Autodesk Inventor part; units mm, degrees
ref_plane "YZ Plane" through (0, 0, 0) normal (1, 0, 0) x (0, 1, 0)
ref_plane "XZ Plane" through (0, 0, 0) normal (0, 1, 0) x (-1, 0, 0)
ref_plane "XY Plane" through (0, 0, 0) normal (0, 0, 1) x (1, 0, 0)
sketch "Sketch1" plane through (0, 0, 0) normal (0, 0, 1) x (1, 0, 0)
  line L0 (-21.2294, -12.5998) -> (21.2706, -12.5998)
  line L1 (23.2706, -10.5998) -> (23.2706, -4.1998)
  line L2 (-23.2294, -4.1998) -> (-23.2294, -10.5998)
  line L3 (12.0206, -0.1998) -> (12.0206, 21.8002)
  line L4 (10.0206, 23.8002) -> (-9.9794, 23.8002)
  line L5 (-11.9794, 21.8002) -> (-11.9794, -0.1998)
  circle A0 centre (16.0206, -7.3998) radius 1.6
  circle A1 centre (-15.9794, -7.3998) radius 1.6
  line L6 (21.2706, -2.1998) -> (14.0206, -2.1998)
  line L7 (-13.9794, -2.1998) -> (-21.2294, -2.1998)
  line L8 (0.0206, 11.8002) -> (-1.5294, 11.8002)
  line L9 (-1.5294, 11.8002) -> (1.5706, 11.8002)
  line L10 (-1.5294, 11.8002) -> (-1.5294, 13.8002)
  line L11 (-1.5294, 13.8002) -> (-2.7282, 13.8002)
  line L12 (2.7718, 13.8002) -> (2.7718, 15.8002)
  line L13 (-2.7282, 15.8002) -> (-2.7282, 13.8002)
  line L14 (-2.7282, 15.8002) -> (-1.5294, 15.8002)
  line L15 (0.0206, 15.8002) -> (0.0218, 15.8002)
  line L16 (2.7718, 15.8002) -> (1.5706, 15.8002)
  line L17 (-1.5294, 15.8002) -> (-2.7282, 15.8002)
  line L18 (-1.5294, 11.8002) -> (-1.5294, 13.8002)
  line L19 (-1.5294, 15.8002) -> (-1.5294, 23.8002)
  line L20 (-2.7282, 13.8002) -> (-1.5294, 13.8002)
  line L21 (1.5706, 13.8002) -> (2.7718, 13.8002)
  line L22 (1.5706, 11.8002) -> (1.5706, 13.8002)
  line L23 (1.5706, 15.8002) -> (1.5706, 23.8002)
  arc A2 (23.2706, -4.1998) -> (21.2706, -2.1998) centre (21.2706, -4.1998) ccw
  arc A3 (21.2706, -12.5998) -> (23.2706, -10.5998) centre (21.2706, -10.5998) ccw
  arc A4 (-23.2294, -10.5998) -> (-21.2294, -12.5998) centre (-21.2294, -10.5998) ccw
  arc A5 (-21.2294, -2.1998) -> (-23.2294, -4.1998) centre (-21.2294, -4.1998) ccw
  arc A6 (-13.9794, -2.1998) -> (-11.9794, -0.1998) centre (-13.9794, -0.1998) ccw
  arc A7 (12.0206, -0.1998) -> (14.0206, -2.1998) centre (14.0206, -0.1998) ccw
  arc A8 (-9.9794, 23.8002) -> (-11.9794, 21.8002) centre (-9.9794, 21.8002) ccw
  arc A9 (12.0206, 21.8002) -> (10.0206, 23.8002) centre (10.0206, 21.8002) ccw
  point P0 (0, 0)
  point P1 (0, 0)
  point P2 (12.0206, 23.8002)
  point P3 (-11.9794, 23.8002)
  dimension "d0" = 24
  dimension "d1" = 3.2
  dimension "d2" = 3.2
  dimension "d3" = 2
extrude "Extrusion1" add sketch "Sketch1" along normal blind 6 contours A4 L2 A5 L7 A6 L5 A8 L4 L19 L14 L13 L11 L10 L8 L9 L22 L21 L12 L16 L23 A9 L3 A7 L6 A2 L1 A3 L0
sketch "Sketch2" plane through (0, 0, 6) normal (0, 0, 1) x (1, 0, 0)
  circle A0 centre (-6.9812, 28.6469) radius 1.6
  circle A1 centre (7.0188, 28.6469) radius 1.6
  circle A2 centre (-17.6062, 13.3479) radius 1.6
  circle A3 centre (17.6438, 13.3479) radius 1.6
  line L0 (-23.2312, 26.8921) -> (-23.2312, -30.3531)
  arc A4 (-23.2312, -30.3531) -> (-21.2312, -32.3531) centre (-21.2312, -30.3531) ccw
  line L1 (-21.2312, -32.3531) -> (-7.8931, -32.3531)
  arc A5 (21.2688, -32.3531) -> (23.2688, -30.3531) centre (21.2688, -30.3531) ccw
  line L2 (23.2688, -30.3531) -> (23.2688, 26.8921)
  arc A6 (23.2688, 26.8921) -> (21.8599, 27.8047) centre (22.2688, 26.8921) ccw
  arc A7 (12.0188, 33.6469) -> (21.8599, 27.8047) centre (18.9975, 34.1927) ccw
  line L3 (12.0188, 33.6469) -> (12.0188, 39.5469)
  arc A8 (12.0188, 39.5469) -> (10.0188, 41.5469) centre (10.0188, 39.5469) ccw
  line L4 (10.0188, 41.5469) -> (2.5188, 41.5469)
  arc A9 (2.5188, 41.5469) -> (1.5188, 40.5469) centre (2.5188, 40.5469) ccw
  line L5 (1.5188, 40.5469) -> (1.5188, 36.5469)
  line L6 (1.5188, 36.5469) -> (2.7688, 36.5469)
  line L7 (2.7688, 36.5469) -> (2.7688, 33.6469)
  line L8 (2.7688, 33.6469) -> (1.5688, 33.6469)
  line L9 (1.5688, 33.6469) -> (1.5688, 23.6469)
  line L10 (1.5688, 23.6469) -> (10.0188, 23.6469)
  arc A10 (12.0188, 21.6469) -> (10.0188, 23.6469) centre (10.0188, 21.6469) ccw
  line L11 (12.0188, 21.6469) -> (12.0188, -0.3531)
  arc A11 (12.0188, -0.3531) -> (14.0188, -2.3531) centre (14.0188, -0.3531) ccw
  line L12 (14.0206, -2.3531) -> (16.2688, -2.3531)
  arc A12 (18.2688, -4.3531) -> (16.2688, -2.3531) centre (16.2688, -4.3531) ccw
  line L13 (18.2688, -4.3531) -> (18.2688, -21.3531)
  arc A13 (16.2688, -23.3531) -> (18.2688, -21.3531) centre (16.2688, -21.3531) ccw
  line L14 (16.2688, -23.3531) -> (-16.2312, -23.3531)
  arc A14 (-18.2312, -21.3531) -> (-16.2312, -23.3531) centre (-16.2312, -21.3531) ccw
  line L15 (-18.2312, -21.3531) -> (-18.2312, -4.3531)
  arc A15 (-16.2312, -2.3531) -> (-18.2312, -4.3531) centre (-16.2312, -4.3531) ccw
  line L16 (-16.2312, -2.3531) -> (-13.9794, -2.3531)
  arc A16 (-13.9794, -2.3531) -> (-11.9812, -0.5065) centre (-13.9753, -0.3531) ccw
  line L17 (-11.9812, -0.5065) -> (-11.9812, 21.4935)
  arc A17 (-9.9812, 23.4935) -> (-11.9812, 21.4935) centre (-9.9812, 21.4935) ccw
  line L18 (-9.9812, 23.4935) -> (-1.5312, 23.4935)
  line L19 (-1.5312, 23.4935) -> (-1.5312, 33.4935)
  line L20 (-1.5312, 33.4935) -> (-2.7312, 33.4935)
  line L21 (-2.7312, 33.4935) -> (-2.7312, 36.3935)
  line L22 (-2.7312, 36.3935) -> (-1.4812, 36.3935)
  line L23 (-1.4812, 36.3935) -> (-1.4812, 40.5469)
  arc A18 (-1.4812, 40.5469) -> (-2.4812, 41.5469) centre (-2.4812, 40.5469) ccw
  line L24 (-2.4812, 41.5469) -> (-9.9812, 41.5469)
  arc A19 (-9.9812, 41.5469) -> (-11.9812, 39.5469) centre (-9.9812, 39.5469) ccw
  line L25 (-11.9812, 39.5469) -> (-11.9812, 33.6469)
  arc A20 (-21.8223, 27.8047) -> (-11.9812, 33.6469) centre (-18.9599, 34.1927) ccw
  arc A21 (-21.8223, 27.8047) -> (-23.2312, 26.8921) centre (-22.2312, 26.8921) ccw
  line L26 (-13.9794, -2.3531) -> (-21.2294, -2.3531)
  arc A22 (-21.2294, -2.3531) -> (-23.2294, -4.3531) centre (-21.2294, -4.3531) ccw
  line L27 (-23.2294, -4.3531) -> (-23.2294, -10.7531)
  arc A23 (-23.2294, -10.7531) -> (-21.2294, -12.7531) centre (-21.2294, -10.7531) ccw
  line L28 (-21.2294, -12.7531) -> (21.2706, -12.7531)
  line L29 (21.2706, -2.3531) -> (14.0206, -2.3531)
  arc A24 (23.2706, -4.3531) -> (21.2706, -2.3531) centre (21.2706, -4.3531) ccw
  line L30 (23.2706, -10.7531) -> (23.2706, -4.3531)
  arc A25 (21.2706, -12.7531) -> (23.2706, -10.7531) centre (21.2706, -10.7531) ccw
  arc A26 (5.9613, -30.7014) -> (7.9307, -32.3531) centre (7.9307, -30.3531) ccw
  line L31 (7.9307, -32.3531) -> (21.2688, -32.3531)
  arc A27 (-7.8931, -32.3531) -> (-5.9236, -30.7014) centre (-7.8931, -30.3531) ccw
  arc A28 (5.9613, -30.7014) -> (-5.9236, -30.7014) centre (0.0188, -31.7522) ccw
  point P0 (0, 0)
  point P1 (-18.2312, -12.7531)
  point P2 (18.2688, -12.7531)
extrude "Extrusion2" cut sketch "Sketch2" against normal blind 6 contours A22 L26 A15 L15 L28 A23 L0 | L13 A12 L29 A24 L2 A25 L28
fillet "Fillet1" radius 2 2 edges at (18.2688, -12.5998, 3) (-18.2312, -12.5998, 3)
sketch "Sketch4" plane through (-1.5294, 11.8002, 0) normal (0, 1, 0) x (1, 0, 0)
  line L0 (3.1, 0) -> (0, 0)
  line L1 (0, 0) -> (0, -6)
  line L2 (3.1, -6) -> (0, -6)
  line L3 (3.1, 0) -> (3.1, -6)
  point P0 (1.5294, 0)
extrude "Extrusion3" cut sketch "Sketch4" against normal blind 13
sketch "Sketch5" plane through (-2.7282, 15.8002, 0) normal (0, -1, 0) x (1, 0, 0)
  line L0 (0, 0) -> (1.1988, 0)
  line L1 (1.1988, 0) -> (1.1988, 6)
  line L2 (0, 6) -> (1.1988, 6)
  line L3 (0, 0) -> (0, 6)
  line L4 (4.2988, 0) -> (5.5, 0)
  line L5 (5.5, 0) -> (5.5, 6)
  line L6 (4.2988, 6) -> (5.5, 6)
  line L7 (4.2988, 0) -> (4.2988, 6)
  point P0 (2.7282, 0)
extrude "Extrusion4" add sketch "Sketch5" along normal blind 0.4
sketch "Sketch6" plane through (0, 0, 6) normal (0, 0, 1) x (1, 0, 0)
  line L0 (22.9743, 18.6641) -> (86.0826, 18.6641) construction
  line L1 (86.0826, 18.6641) -> (86.0826, -0.0954) construction
  line L2 (86.0826, -0.0954) -> (22.9743, -0.0954) construction
  line L3 (22.9743, -0.0954) -> (22.9743, 18.6641) construction
  point P0 (0, 0)
extrude "Extrusion5" [suppressed]
properties part number "Hotend Slide Part 1"
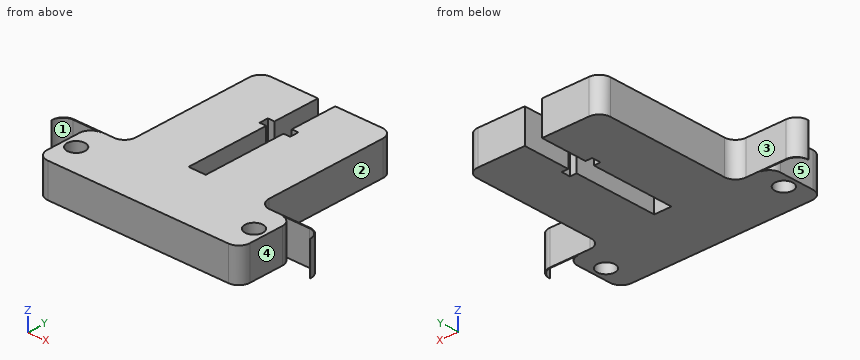
Check sheet for the modelled part. Datum: model origin and axes. Units: mm. Face numbers are marked on the shaded views. A direction names the side the tool comes from. Round coordinates to 2 decimals unless told otherwise and drop trailing zeros. Loops run counter-clockwise (first coordinate to the right, second up) from the corner with the lowest first, then second, coordinate; pieces in that order, holes last. Notation, with made-up numbers: M 10.5,13 L 63.5,13 A22 cw 63.5,28 Z; hole C 76,62.5 d5. An arc over 180 degrees is marked long. Answer as a JSON object with one key per item and string values.
1. Scan lines: line 1 (X direction, y = -7.5, z = 1.9); line 2 (X direction, y = 8, z = 4.65); line 3 (X direction, y = 14, z = 4). Record each from-to range of solid material in increasing order.
Reply:
{"line 1": "x = -18.23 to -17.58, -14.38 to 14.42, 17.62 to 18.27", "line 2": "x = -11.98 to -1.53, 1.57 to 12.02", "line 3": "x = -11.98 to -2.73, 2.77 to 12.02"}
2. Section check D-D (x = -1). Record the boundary of the cut face in (y, z).
Reply:
{"outline": "M -12.6,0 L -1.2,0 L -1.2,6 L -12.6,6 Z"}
3. Section check C-C (y = 14.5). Record the boundary of the cut face in (x, z).
Reply:
{"outline": "M -11.98,0 L -2.73,0 L -2.73,6 L -11.98,6 Z; M 2.77,0 L 12.02,0 L 12.02,6 L 2.77,6 Z"}
4. Section check B-B (y = -8). Record the boundary of the cut face in (x, z), plus the area to 3 significant figures.
Reply:
{"outline": "M -18.23,0 L -17.46,0 L -17.46,6 L -18.23,6 Z; M -14.5,0 L 14.54,0 L 14.54,6 L -14.5,6 Z; M 17.5,0 L 18.27,0 L 18.27,6 L 17.5,6 Z", "area": "183 mm²"}
5. Section check A-A (y = 3.5). Record the boundary of the cut face in (x, z), plus the area to 3 significant figures.
Reply:
{"outline": "M -11.98,0 L -1.53,0 L -1.53,6 L -11.98,6 Z; M 1.57,0 L 12.02,0 L 12.02,6 L 1.57,6 Z", "area": "125 mm²"}
6. Gauge pin test, flat ends, axial feed: P1, Ø0.5, axis at y = 15, z = 3.5, coming from the -X side; P2, Ø1.3, axis at y = 14, z = 3.5, coming from the +X side; P3, Ø2, axis at x = 15, y = 6.5, coming from the +Z side; P4, Ø1.5, axis at y = -2.5, z = 2.5, coming from the -X side. Record the tip position at first contact, or that the pin passes through.
Reply:
{"P1": "stops at x = -11.98", "P2": "stops at x = 12.02", "P3": "passes through", "P4": "stops at x = -22.99"}
7. Access from +Z, -Z, +X, -X, +Y, -Y to the whole of each face (thin tool, end or side, straight path). Record for the marked faces 1, 2, 3, 4 and 5.
Reply:
{"face 1": "+Z, -Z, -Y", "face 2": "+Z, -Z, +X, +Y", "face 3": "+Z, -Z, -X, +Y", "face 4": "+Z, -Z, +X, -Y", "face 5": "+Z, -Z, -X, -Y"}
